```python
from build123d import *

# Parameters (mm, degrees)
SKETCH_1_W             = 15
SKETCH_1_H             = 50
EXTRUDE_1_DEPTH        = 3
SKETCH_2_W             = 15
SKETCH_2_H             = 4.5
EXTRUDE_2_DEPTH        = 12
SKETCH_3_W             = 15
SKETCH_3_H             = 50
SKETCH_3_W_2           = 11
SKETCH_3_H_2           = 41
EXTRUDE_3_DEPTH        = 3
EXTRUDE_4_DEPTH        = 3
HOLE_WIZARD_M3_1_D     = 2.5
HOLE_WIZARD_M3_1_DEPTH = 3
CUT_EXTRUDE_1_REACH    = 23
SKETCH_8_W             = 3
SKETCH_8_H             = 50
HOLE_WIZARD_M3_2_D     = 2.5
HOLE_WIZARD_M3_2_DEPTH = 10
HOLE_WIZARD_M3_2_TIP   = 0.751075774


with BuildPart() as part:
    # 스케치1 → 보스-돌출1 (new body)
    with BuildSketch(Plane.XY):
        Rectangle(SKETCH_1_W, SKETCH_1_H)
    extrude(amount=EXTRUDE_1_DEPTH)

    # 스케치2 → 보스-돌출2 (add)
    with BuildSketch(Plane(origin=(0, 0, 0), x_dir=(-1, 0, 0), z_dir=(0, 0, -1))):
        with Locations((0, 22.75)):
            Rectangle(SKETCH_2_W, SKETCH_2_H)
        with Locations((0, -22.75)):
            Rectangle(SKETCH_2_W, SKETCH_2_H)
    extrude(amount=EXTRUDE_2_DEPTH)

    # 스케치3 → 보스-돌출3 (add)
    with BuildSketch(Plane(origin=(0, 0, -12), x_dir=(-1, 0, 0), z_dir=(0, 0, -1))):
        Rectangle(SKETCH_3_W, SKETCH_3_H)
        Rectangle(SKETCH_3_W_2, SKETCH_3_H_2, mode=Mode.SUBTRACT)
    extrude(amount=EXTRUDE_3_DEPTH)

    # 스케치5 → 보스-돌출4 (add)
    with BuildSketch(Plane(origin=(0, 0, -15), x_dir=(-1, 0, 0), z_dir=(0, 0, -1))):
        Polygon((-7.5, 16.5), (-10.5, 16.5), (-10.5, 18.5), (-13.5, 18.5), (-13.5, 10.5), (-10.5, 10.5), (-10.5, 12.5), (-7.5, 12.5), align=None)
        Polygon((7.5, 16.5), (7.5, 12.5), (10.5, 12.5), (10.5, 10.5), (13.5, 10.5), (13.5, 18.5), (10.5, 18.5), (10.5, 16.5), align=None)
        Polygon((7.5, -16.5), (10.5, -16.5), (10.5, -18.5), (13.5, -18.5), (13.5, -10.5), (10.5, -10.5), (10.5, -12.5), (7.5, -12.5), align=None)
        Polygon((-7.5, -16.5), (-7.5, -12.5), (-10.5, -12.5), (-10.5, -10.5), (-13.5, -10.5), (-13.5, -18.5), (-10.5, -18.5), (-10.5, -16.5), align=None)
    extrude(amount=-EXTRUDE_4_DEPTH)

    # M3 나사 구멍1
    with Locations(Plane.XY.offset(3)):
        with Locations((0, 5), (0, -5)):
            Hole(HOLE_WIZARD_M3_1_D / 2, depth=HOLE_WIZARD_M3_1_DEPTH)

    # 스케치8 → 컷-돌출1 (cut, up to next)
    with BuildSketch(Plane.ZY.offset(7.5), mode=Mode.PRIVATE) as cut_extrude_1_sk1:
        with Locations((1.5, 0)):
            Rectangle(SKETCH_8_W, SKETCH_8_H)
    cut_extrude_1_tool1 = extrude(cut_extrude_1_sk1.sketch, amount=-CUT_EXTRUDE_1_REACH, mode=Mode.PRIVATE) & part.part
    add(cut_extrude_1_tool1.solids().sort_by_distance((-7.5, 0, 1.5))[0], mode=Mode.SUBTRACT)

    # M3 나사 구멍2
    with Locations(Plane.XY):
        with Locations((-5, 22.5), (5, 22.5), (-5, -22.5), (5, -22.5)):
            Hole(HOLE_WIZARD_M3_2_D / 2, depth=HOLE_WIZARD_M3_2_DEPTH)
            with Locations((0, 0, -(HOLE_WIZARD_M3_2_DEPTH + HOLE_WIZARD_M3_2_TIP / 2))):  # 118° drill point
                Cone(0, HOLE_WIZARD_M3_2_D / 2, HOLE_WIZARD_M3_2_TIP, mode=Mode.SUBTRACT)


solid = part.part
```
CAD build for the part. Positions are in the model's coordinates, mm. A direction names the side the tool comes from. Round coordinates to 2 decimals unless told otherwise and drop trailing zeros. Write each loop counter-clockwise with the first axis right and the second up, starting at its lowest first coordinate (ties: lowest second). Pieces come first, ordered by that corner, then holes.
Item 1: Band-saw the part on A-A on z = -2.5. Write the cut outline in (x, y).
Filled in:
outline: (-7.5, -25) - (7.5, -25) - (7.5, -20.5) - (-7.5, -20.5) - close; (-7.5, 20.5) - (7.5, 20.5) - (7.5, 25) - (-7.5, 25) - close; hole circle Ø2.5 at (-5, -22.5); hole circle Ø2.5 at (-5, 22.5); hole circle Ø2.5 at (5, -22.5); hole circle Ø2.5 at (5, 22.5)
Item 2: Drop flat-ended pins along their axis: pin 1 Ø1.5 at (x, z) = (11.5, -13.5) entering from -Y; pin 2 Ø2.5 at (x, z) = (-9, -14) entering from -Y; pin 3 Ø4 at (x, y) = (5, -5) entering from +Z. Give the stop position or say it passes through.
Filled in:
pin 1: stops at y = -18.5
pin 2: stops at y = -16.5
pin 3: stops at z = -12
Item 3: Mould opens along Y. For faces 6 (the flat face through (7.5, 0, -13)), 7 (the flat face through (-13.5, -15, -14)), 8 (the flat face through (9, -16.5, -14)) say: released by +Y, released by -Y, zero draft, split by the parting line, or undercut.
Filled in:
face 6: undercut
face 7: zero draft
face 8: released by -Y
Item 4: Drill centre lines: L1, parallel to X at y = 22.5, z = -6.75; L2, parallel to Y at x = 5, z = -5; L3, parallel to Y at x = -3.25, z = -3. Where is each one in solid material? Low to high.
Filled in:
L1: x = -7.5 to -6.25, -3.75 to 3.75, 6.25 to 7.5
L2: y = -25 to -23.75, -21.25 to -20.5, 20.5 to 21.25, 23.75 to 25
L3: y = -25 to -20.5, 20.5 to 25
Item 5: Band-saw the part on C-C on y = -5. Write the cut outline in (x, z).
Filled in:
outline: (-7.5, -15) - (-5.5, -15) - (-5.5, -12) - (-7.5, -12) - close; (5.5, -15) - (7.5, -15) - (7.5, -12) - (5.5, -12) - close
Item 6: Tool access for faces 1 (the flat face through (-10.5, 18, -14)), 2 (the cylindrical face through (-4.73, 21.28, -5.07)), 3 (the flat face through (10.5, -12, -14)), 4 (the flat face through (-12, -10.5, -14)), 5 (the flat face through (7, 0, -12)): list every direction of +Z, -Z, +X, -X, +Y, -Y with a clear straight run to the whole face (end or side of a thin tool).
Filled in:
face 1: +Z, -Z, +Y
face 2: +Z
face 3: +Z, -Z
face 4: +Z, -Z, -X
face 5: +Z, +X, -X
Item 7: Band-saw the part on B-B on x = 11.25. Write the cut outline in (y, z), then the cut area to 3 significant figures.
Filled in:
outline: (-18.5, -15) - (-10.5, -15) - (-10.5, -12) - (-18.5, -12) - close; (10.5, -15) - (18.5, -15) - (18.5, -12) - (10.5, -12) - close
area: 48.0 mm2
